Part model, mm, in its own coordinate system. A direction names the side the tool comes from. Round coordinates to 2 decimals unless told otherwise and drop trailing zeros. Write each loop counter-clockwise with the first axis right and the second up, starting at its lowest first coordinate (ties: lowest second). Pieces come first, ordered by that corner, then holes.
Autodesk Inventor part; units mm, degrees
ref_plane "YZ Plane" through (0, 0, 0) normal (1, 0, 0) x (0, 1, 0)
ref_plane "XZ Plane" through (0, 0, 0) normal (0, 1, 0) x (-1, 0, 0)
ref_plane "XY Plane" through (0, 0, 0) normal (0, 0, 1) x (1, 0, 0)
sketch "Sketch1" plane through (0, 0, 0) normal (1, 0, 0) x (0, 1, 0)
  line L0 (-6, -12.5) -> (-6, -12.9)
  arc A0 (-6, -12.9) -> (-5.6, -13.3) centre (-5.6, -12.9) ccw
  line L1 (-5.6, -13.3) -> (-4.9, -13.3)
  arc A1 (-4.9, -13.3) -> (-4.7, -13.1) centre (-4.9, -13.1) ccw
  line L2 (-4.7, -13.1) -> (-4.7, -12.85)
  arc A2 (-4.5, -12.65) -> (-4.7, -12.85) centre (-4.5, -12.85) ccw
  line L3 (-4.5, -12.65) -> (-1.8, -12.65)
  arc A3 (-1.4, -13.05) -> (-1.8, -12.65) centre (-1.8, -13.05) ccw
  line L4 (-1.4, -13.05) -> (-1.4, -18.75)
  line L5 (-1.8, -19.15) -> (-4.5, -19.15)
  arc A4 (-1.8, -19.15) -> (-1.4, -18.75) centre (-1.8, -18.75) ccw
  arc A5 (-4.7, -18.95) -> (-4.5, -19.15) centre (-4.5, -18.95) ccw
  line L6 (-4.7, -18.95) -> (-4.7, -18.7)
  arc A6 (-4.7, -18.7) -> (-4.9, -18.5) centre (-4.9, -18.7) ccw
  line L7 (-4.9, -18.5) -> (-5.6, -18.5)
  arc A7 (-5.6, -18.5) -> (-6, -18.9) centre (-5.6, -18.9) ccw
  line L8 (-6, -18.9) -> (-6, -19.5)
  line L9 (-6.5, -6.5) -> (-6.5, -12.5)
  line L10 (-6.5, -12.5) -> (-2.5, -12.5)
  line L11 (-1.05, -19.5) -> (-6.5, -19.5)
  line L12 (-6.5, -19.5) -> (-6.5, -26)
  line L13 (-6.5, -26) -> (-1.05, -26)
  line L14 (-6, -26) -> (-6, -26.6)
  arc A8 (-6, -26.6) -> (-5.6, -27) centre (-5.6, -26.6) ccw
  line L15 (-5.6, -27) -> (-4.9, -27)
  arc A9 (-4.9, -27) -> (-4.7, -26.8) centre (-4.9, -26.8) ccw
  arc A10 (-4.5, -26.35) -> (-4.7, -26.55) centre (-4.5, -26.55) ccw
  line L16 (-4.7, -26.8) -> (-4.7, -26.55)
  line L17 (-4.5, -26.35) -> (-1.8, -26.35)
  arc A11 (-1.4, -26.75) -> (-1.8, -26.35) centre (-1.8, -26.75) ccw
  line L18 (-1.4, -26.75) -> (-1.4, -32.45)
  arc A12 (-1.8, -32.85) -> (-1.4, -32.45) centre (-1.8, -32.45) ccw
  line L19 (-1.8, -32.85) -> (-4.5, -32.85)
  arc A13 (-4.7, -32.65) -> (-4.5, -32.85) centre (-4.5, -32.65) ccw
  line L20 (-4.7, -32.65) -> (-4.7, -32.4)
  arc A14 (-4.7, -32.4) -> (-4.9, -32.2) centre (-4.9, -32.4) ccw
  line L21 (-4.9, -32.2) -> (-5.6, -32.2)
  arc A15 (-5.6, -32.2) -> (-6, -32.6) centre (-5.6, -32.6) ccw
  line L22 (-6, -32.6) -> (-6, -33)
  line L23 (-2.5, -33) -> (-6.5, -33)
  line L24 (-6.5, -33) -> (-6.5, -39)
  line L25 (32.5, 0) -> (0, 0)
  circle A16 centre (0, -6.5) radius 4.75
  circle A17 centre (32.5, -6.5) radius 4.75
  circle A18 centre (0, -39) radius 4.75
  circle A19 centre (32.5, -39) radius 4.75
  line L26 (39, -26) -> (39, -19.5)
  line L27 (39, -12.5) -> (39, -6.5)
  line L28 (39, -39) -> (39, -33)
  line L29 (26.5, -45.5) -> (32.5, -45.5)
  line L30 (0, -45.5) -> (6, -45.5)
  line L31 (13, -45.5) -> (19.5, -45.5)
  circle A20 centre (16.25, -22.75) radius 15
  circle A21 centre (16.2588, 5.0016) radius 2.5
  circle A22 centre (16.25, -50.5) radius 2.5
  circle A23 centre (16.25, -22.75) radius 5
  circle A24 centre (16.25, -22.75) radius 8.45
  line L32 (24.75, -27.6575) -> (24.75, -17.8425)
  line L33 (44, 10) -> (-11.5, 10)
  line L34 (-11.5, 10) -> (-11.5, -55.5)
  line L35 (-11.5, -55.5) -> (44, -55.5)
  line L36 (44, -55.5) -> (44, 10)
  line L37 (-11.5, 30) -> (44, 30)
  line L38 (-11.5, -75.5) -> (-11.5, 30)
  line L39 (44, 30) -> (44, -75.5)
  line L40 (44, -75.5) -> (-11.5, -75.5)
  circle A25 centre (16.25, -65.5) radius 5
  circle A26 centre (16.25, 20) radius 5
  arc A27 (39, -6.5) -> (32.5, 0) centre (32.5, -6.5) ccw
  arc A28 (32.5, -45.5) -> (39, -39) centre (32.5, -39) ccw
  arc A29 (0, 0) -> (-6.5, -6.5) centre (0, -6.5) ccw
  arc A30 (-6.5, -39) -> (0, -45.5) centre (0, -39) ccw
  line L41 (39, -12.5) -> (39, -33)
  line L42 (26.5, -45.5) -> (6, -45.5)
  line L43 (-6.5, -12.5) -> (-6.5, -33)
extrude "Extrusion1" add sketch "Sketch1" along normal blind 5 contours L10 L9 A29 L25 A27 L27 L41 L26 L28 A28 L29 L42 L31 L30 A30 L24 L23 L22 A15 L21 A14 L20 A13 L19 A12 L18 A11 L17 A10 L16 A9 L15 A8 L14 L13 L12 L11 L8 A7 L7 A6 L6 A5 L5 A4 L4 A3 L3 A2 L2 A1 L1 A0 L0 | L0 A0 L1 A1 L2 A2 L3 A3 L4 A4 L5 A5 L6 A6 L7 A7 L8 L11 L43 L10 | L13 L14 A8 L15 A9 L16 A10 L17 A11 L18 A12 L19 A13 L20 A14 L21 A15 L22 L23 L43 | A20 | A23 | A24
sketch "Sketch2" plane through (5, 0, 0) normal (1, 0, 0) x (0, 0, -1)
  circle A0 centre (6.5, 32.5) radius 4.75
  circle A1 centre (39, 0) radius 4.75
  line L0 (6.5, 32.5) -> (39, 0)
  circle A2 centre (39, 32.5) radius 4.75
  line L1 (39, 0) -> (39, 32.5)
  line L2 (39, 32.5) -> (6.5, 0)
  circle A3 centre (22.75, 16.25) radius 5
  circle A4 centre (22.75, 16.25) radius 10
  point P0 (0, 0)
  dimension "d2" = 10
  dimension "d3" = 20
extrude "Extrusion2" add sketch "Sketch2" along normal blind 13 contours A4 L2 A3 L0 | L0 A3 L2 A4 | A4 L0 A3 L2 | L2 A3 L0 A4
fillet "Fillet1" radius 5 1 edges at (5, 16.25, -12.75)
properties part number "CodoHidráulicos"
Q1. Drop flat-ended pins along their axis: pin 1 (1 mm diameter, centred on y = 33, z = -33.5, fed in from -X); pin 2 (5 mm diameter, centred on y = 18, z = -24, fed in from +X); pin 3 (8.5 mm diameter, centred on y = 32.5, z = -39, fed in from -X); pin 4 (2 mm diameter, centred on x = 10.5, z = -26, fed in from -Y). Give the stop position or say it passes through.
Values follow:
pin 1: stops at x = 0
pin 2: stops at x = 5
pin 3: passes through
pin 4: stops at y = 6.51
Q2. Cut at A-A on x = 2. Write the cut outline in (y, z).
Values follow:
outline: (-6.5, -39) arc R6.5 ccw to (0, -45.5) - (32.5, -45.5) arc R6.5 ccw to (39, -39) - (39, -6.5) arc R6.5 ccw to (32.5, 0) - (0, 0) arc R6.5 ccw to (-6.5, -6.5) - close; hole circle Ø9.5 at (0, -39); hole circle Ø9.5 at (0, -6.5); hole circle Ø9.5 at (32.5, -39); hole circle Ø9.5 at (32.5, -6.5)
Q3. Cut at D-D on z = -22.75. Write the cut outline in (x, y), plus the area to 3 significant figures.
Values follow:
outline: (0, -6.5) - (5, -6.5) - (5, 1.25) arc R5 cw to (10, 6.25) - (18, 6.25) - (18, 11.25) - (5, 11.25) - (5, 21.25) - (18, 21.25) - (18, 26.25) - (10, 26.25) arc R5 cw to (5, 31.25) - (5, 39) - (0, 39) - close
area: 368 mm2
Q4. Wall check: L1, parallel to Z at x = 3.5, y = 32.5; L2, parallel to Z at x = 9.75, y = 16.25; L3, parallel to Y at x = 9.75, z = -22.75. Give the ranges that are in metal, low to high.
Values follow:
L1: z = -45.5 to -43.75, -34.25 to -11.25, -1.75 to 0
L2: z = -32.76 to -27.75, -17.75 to -12.74
L3: y = 6.24 to 11.25, 21.25 to 26.26
Q5. Cut at C-C on y = 16.25. Write the cut outline in (x, z), plus the area to 3 significant figures.
Values follow:
outline: (0, -45.5) - (5, -45.5) - (5, -37.75) arc R5 cw to (10, -32.75) - (18, -32.75) - (18, -27.75) - (5, -27.75) - (5, -17.75) - (18, -17.75) - (18, -12.75) - (10, -12.75) arc R5 cw to (5, -7.75) - (5, 0) - (0, 0) - close
area: 368 mm2
Q6. Cut at B-B on y = 34. Write the cut outline in (x, z), plus the area to 3 significant figures.
Values follow:
outline: (0, -45.32) - (5, -45.32) - (5, -43.51) - (0, -43.51) - close; (0, -34.49) - (5, -34.49) - (5, -11.01) - (0, -11.01) - close; (0, -1.99) - (5, -1.99) - (5, -0.18) - (0, -0.18) - close
area: 136 mm2
Q7. Mould opens along Z. For faces 1 (the flat face through (2, 16, 0)), 2 (the flat face through (5, 16, -23)), 3 (the flat face through (2, 39, -23)) say: +Z half, -Z half, draft (parallel to the pull), parting line (faces both ways), or undercut.
Values follow:
face 1: +Z half
face 2: undercut
face 3: draft
Q8. Which spindle directions (+Z, -Z, +X, -X, +Y, -Y) get a long thin tool onto all of the face, cutting with end or side? Do faces 4 (the flat face through (18, 14, -18)), 5 (the cylindrical face through (11.41, 19.29, -18.78)). Say none if no direction does.
Values follow:
face 4: +Z, -Z, +X, +Y, -Y
face 5: +X
